Verification items for this drawing (mm, ordinates from the low corner). Give positions to 0.01 mm unless a question says otherwise; leave off trailing zeros. Loops run counter-clockwise (first coordinate to the right, second up) from the corner with the lowest first, then second, coordinate; pieces in that order, holes last. Notation, with made-up numbers: (-36.75, 15.5) -> (-32.75, 15.5) arc R30 ccw to (-32.75, 41.5) -> close; hole circle Ø6 at (50, 52.25). An arc over 180 degrees is marked (long way). Answer as a JSON object with one key per item and string values.
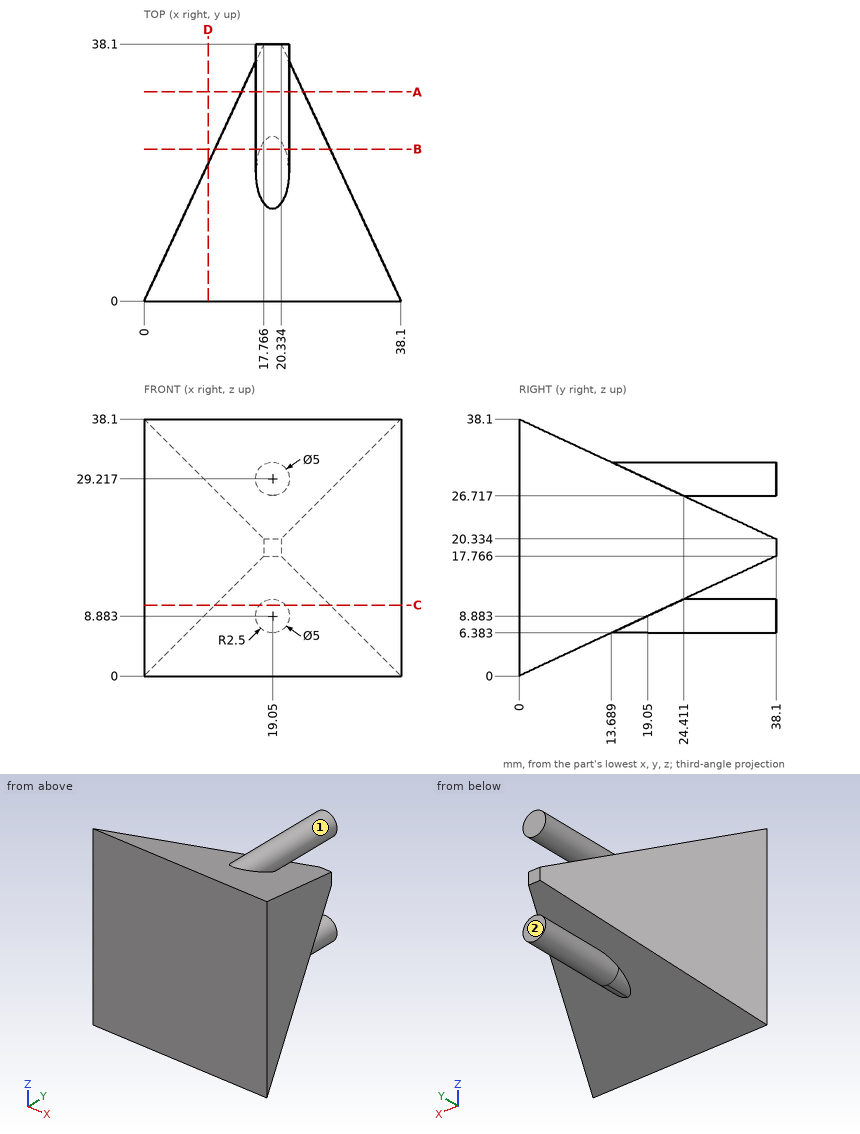
1) Section check C-C on z = 10.5. Record the cut outline in (x, y).
Geometry check:
{"outline": "(0, 0) -> (38.1, 0) -> (27.6, 22.52) -> (20.96, 22.52) -> (20.96, 38.1) -> (17.14, 38.1) -> (17.14, 22.52) -> (10.5, 22.52) -> close"}
2) Section check B-B on y = 22.5. Record the cut outline in (x, z).
Geometry check:
{"outline": "(10.49, 10.49) -> (17.14, 10.49) arc R2.5 ccw (long way) to (20.96, 10.49) -> (27.61, 10.49) -> (27.61, 27.61) -> (20.96, 27.61) arc R2.5 ccw (long way) to (17.14, 27.61) -> (10.49, 27.61) -> close"}
3) Section check A-A on y = 31. Count the separate pieces of the cut face and the enclosed holes in it, plus the area to 3 significant figures.
Geometry check:
{"separate pieces": "3", "enclosed holes": "0", "area": "124 mm2"}
4) Section check D-D on x = 9.5. Record the cut outline in (y, z), plus the area to 3 significant figures.
Geometry check:
{"outline": "(0, 0) -> (20.37, 9.5) -> (20.37, 28.6) -> (0, 38.1) -> close", "area": "583 mm2"}
5) Draft check along Z on the marked faces 1 and 2. Enter one of: pulls with the +Z half, pulls with the -Z half, needs draft (parallel to the pull), parting line crosses it, or undercut.
Geometry check:
{"face 1": "undercut", "face 2": "needs draft"}
6) Depth check by flat-ended pin: P1, Ø1.5, axis at y = 5.5, z = 11.5, coming from the +X side (1 decimal); P2, Ø8, axis at x = 27.5, z = 25, coming from the +Y side (1 decimal); P3, Ø1.5, axis at x = 25.5, y = 23.5, coming from the -Z side. Enter the tip coordinate at first touch or a pass-through.
Geometry check:
{"P1": "stops at x = 35.9", "P2": "stops at y = 30.9", "P3": "stops at z = 10.61"}
7) Material ranges on line 1 along Y through (x, z) = (7, 14.5); line 2 along Z through (x, y) = (8, 7) (1 decimal); line 3 along Y through (x, z) = (16, 25) (1 decimal), recorded low to high. Write a range as from..to.
Geometry check:
{"line 1": "y = 0..15.01", "line 2": "z = 3.3..34.8", "line 3": "y = 0..28.1"}
